Source: CAD feature listing. Evaluate the final solid. Frame: model axes, mm. A direction names the side the tool comes from. Coordinates: 2 decimals unless noted, no trailing zeros. Order: outer loops, then holes, each group sorted by start corner. A loop starts at its lowest first (then second) coordinate and runs counter-clockwise, first axis right, second up.
```python
from build123d import *

# Parameters (mm, degrees)
F0_W           = 100
F0_H           = 8
F1_DEPTH       = 15
F3_DEPTH       = 8
F5_DEPTH       = 3
F7_D           = 3.4
F7_DEPTH       = 15
F7_CBORE_D     = 6.5
F7_CBORE_DEPTH = 3
F7_TIP         = 1.0214630523
F8_R           = 2


# Not quite as in the source:
# - a feature names something its author has since deleted; it is built from what else it names


with BuildPart() as f1:
    # F0 (on Top) → F1 (new body)
    with BuildSketch(Plane.XY):
        with Locations((50, 4)):
            Rectangle(F0_W, F0_H)
    extrude(amount=F1_DEPTH)

    # F2 (on face) → F3 (cut, through all)
    with BuildSketch(Plane.XZ):
        Polygon((70, 5), (22, 0), (100, 0), (100, 5), align=None)
        with BuildLine():
            Line((0, 6.5), (7.1010205144, 6.5))
            ThreePointArc((7.1010205144, 6.5), (17, 7.5), (7.1010205144, 8.5))
            Line((7.1010205144, 8.5), (0, 8.5))
            Line((0, 8.5), (0, 6.5))
        make_face()
        Polygon((100, 15), (22, 15), (70, 10), (100, 10), align=None)
    extrude(amount=-F3_DEPTH, mode=Mode.SUBTRACT)

    # F4 (on face) → F5 (cut)
    with BuildSketch(Plane(origin=(0, 0, 0), x_dir=(1, 0, 0), z_dir=(0, 0, -1))):
        Polygon((4, -7.4641016151), (7, -5.7320508076), (7, -2.2679491924), (4, -0.5358983849), (1, -2.2679491924), (1, -5.7320508076), align=None)
    extrude(amount=-F5_DEPTH, mode=Mode.SUBTRACT)

    # F7
    with Locations(Plane.XY.offset(15)):
        with Locations((4, 4)):
            CounterBoreHole(F7_D / 2, F7_CBORE_D / 2, F7_CBORE_DEPTH, depth=F7_DEPTH)
            with Locations((0, 0, -(F7_DEPTH + F7_TIP / 2))):  # 118° drill point
                Cone(0, F7_D / 2, F7_TIP, mode=Mode.SUBTRACT)

    # F8
    f8_edges = [f1.edges().sort_by_distance(p)[0] for p in [
        (100, 4, 10),
        (100, 4, 5),
        (70, 4, 5),
        (70, 4, 10),
        (22, 4, 15),
        (22, 4, 0),
    ]]
    fillet(f8_edges, radius=F8_R)


solid = f1.part
```
1. Pin query (flat end, axial travel): P1, Ø2, axis at x = 4.5, y = 2.5, coming from the +Z side; P2, Ø3.5, axis at x = 4.5, y = 4.5, coming from the -Z side; P3, Ø2.5, axis at x = 90, y = 4, coming from the -Z side; P4, Ø3, axis at x = 4, y = 4, coming from the +Z side. Return the tip coordinate at first contact, or that it passes through.
Findings:
P1: stops at z = 12
P2: stops at z = 3
P3: stops at z = 5
P4: passes through
2. Section query A-A on y = 4. Count the separate pieces of the cut face and the enclosed holes in it, plus the area to 3 significant figures.
Findings:
separate pieces: 3
enclosed holes: 0
area: 804 mm2
3. Section query C-C on z = 1.25. Return loops of the section in (x, y).
Findings:
outline: (0, 0) - (34, 0) - (34, 8) - (0, 8) - close; hole (1, 2.27) - (4, 0.54) - (7, 2.27) - (7, 5.73) - (4, 7.46) - (1, 5.73) - close
4. Access query for faces 5 (the face through (2, 4, 6.5)), 6 (the face through (1, 4, 1)), 7 (the face through (84, 4, 5)), 8 (the face through (84, 4, 10)). Directions: +Z, -Z, +X, -X, +Y, -Y. A direction counts if a zero-diameter tool reaches every point of the face in a straight line with its end or side. Return the directions, or none.
Findings:
face 5: -X, +Y, -Y
face 6: -Z
face 7: -Z, +X, +Y, -Y
face 8: +Z, +X, +Y, -Y
5. Draft query along Z for faces 1 (the face through (2, 4, 8.5)), 2 (the face through (46.335, 3.944, 2.535)), 3 (the face through (16.996, 3.944, 7.294)), 4 (the face through (45.665, 3.944, 12.535)). Return one class per face: released by +Z, released by -Z, zero draft, split by the parting line, or undercut.
Findings:
face 1: undercut
face 2: released by -Z
face 3: undercut
face 4: released by +Z
6. Section query B-B on x = 9. Return loops of the section in (y, z).
Findings:
outline: (0, 0) - (8, 0) - (8, 3.5) - (0, 3.5) - close; (0, 11.5) - (8, 11.5) - (8, 15) - (0, 15) - close
7. Ray query, line 1 (Y direction, x = 4, z = 13); line 2 (Y direction, x = 4, z = 5.05); line 3 (X direction, y = 5.5, z = 7.25). Return the intervals inside material, ascending.
Findings:
line 1: y = 0 to 0.75, 7.25 to 8
line 2: y = 0 to 2.3, 5.7 to 8
line 3: x = 16.99 to 100
8. Section query D-D on x = 75.5. Return loops of the section in (y, z), plus the area to 3 significant figures.
Findings:
outline: (0, 5) - (8, 5) - (8, 10) - (0, 10) - close
area: 40.0 mm2
